from build123d import *

# Parameters (mm, degrees)
SKETCH_2_R      = 2.55
SKETCH_2_W      = 14
SKETCH_2_H      = 14
SKETCH_2_W_2    = 50
SKETCH_2_H_2    = 8
EXTRUDE_1_DEPTH = 5


with BuildPart() as part:
    # 草图2 → 凸台-拉伸1 (new body)
    with BuildSketch(Plane.XY):
        with BuildLine():
            Line((-130, 29.5), (130, 29.5))
            ThreePointArc((130, 29.5), (143.788582233, 23.788582233), (149.5, 10))
            Line((149.5, 10), (149.5, -110))
            ThreePointArc((149.5, -110), (143.788582233, -123.788582233), (130, -129.5))
            Line((130, -129.5), (-130, -129.5))
            ThreePointArc((-130, -129.5), (-143.788582233, -123.788582233), (-149.5, -110))
            Line((-149.5, -110), (-149.5, 10))
            ThreePointArc((-149.5, 10), (-143.788582233, 23.788582233), (-130, 29.5))
        make_face()
        with Locations((130, -110)):
            Circle(SKETCH_2_R, mode=Mode.SUBTRACT)
        with Locations((130, 10)):
            Circle(SKETCH_2_R, mode=Mode.SUBTRACT)
        with Locations((-130, -110)):
            Circle(SKETCH_2_R, mode=Mode.SUBTRACT)
        with Locations((-130, 10)):
            Circle(SKETCH_2_R, mode=Mode.SUBTRACT)
        with Locations((-61, -50)):
            Rectangle(SKETCH_2_W, SKETCH_2_H, mode=Mode.SUBTRACT)
        with Locations((-24, -50)):
            Rectangle(SKETCH_2_W, SKETCH_2_H, mode=Mode.SUBTRACT)
        with Locations((24, -50)):
            Rectangle(SKETCH_2_W, SKETCH_2_H, mode=Mode.SUBTRACT)
        with Locations((136, -87)):
            Rectangle(SKETCH_2_W, SKETCH_2_H, mode=Mode.SUBTRACT)
        with Locations((136, -13)):
            Rectangle(SKETCH_2_W, SKETCH_2_H, mode=Mode.SUBTRACT)
        with Locations((0, 6)):
            Rectangle(SKETCH_2_W_2, SKETCH_2_H_2, mode=Mode.SUBTRACT)
        with Locations((-136, -87)):
            Rectangle(SKETCH_2_W, SKETCH_2_H, mode=Mode.SUBTRACT)
        with Locations((-136, -13)):
            Rectangle(SKETCH_2_W, SKETCH_2_H, mode=Mode.SUBTRACT)
        with Locations((-98, -50)):
            Rectangle(SKETCH_2_W, SKETCH_2_H, mode=Mode.SUBTRACT)
        with Locations((61, -50)):
            Rectangle(SKETCH_2_W, SKETCH_2_H, mode=Mode.SUBTRACT)
        with Locations((98, -50)):
            Rectangle(SKETCH_2_W, SKETCH_2_H, mode=Mode.SUBTRACT)
        with BuildLine():
            Line((133.05, -25.838987573), (133.05, -30.161012427))
            ThreePointArc((133.05, -30.161012427), (132, -31.211012427), (130.95, -30.161012427))
            Line((130.95, -30.161012427), (130.95, -25.838987573))
            ThreePointArc((130.95, -25.838987573), (132, -24.788987573), (133.05, -25.838987573))
        make_face(mode=Mode.SUBTRACT)
        with BuildLine():
            Line((141.05, -26), (141.05, -30))
            ThreePointArc((141.05, -30), (140, -31.05), (138.95, -30))
            Line((138.95, -30), (138.95, -26))
            ThreePointArc((138.95, -26), (140, -24.95), (141.05, -26))
        make_face(mode=Mode.SUBTRACT)
        with BuildLine():
            Line((130.95, -74), (130.95, -70))
            ThreePointArc((130.95, -70), (132, -68.95), (133.05, -70))
            Line((133.05, -70), (133.05, -74))
            ThreePointArc((133.05, -74), (132, -75.05), (130.95, -74))
        make_face(mode=Mode.SUBTRACT)
        with BuildLine():
            Line((138.95, -74), (138.95, -70))
            ThreePointArc((138.95, -70), (140, -68.95), (141.05, -70))
            Line((141.05, -70), (141.05, -74))
            ThreePointArc((141.05, -74), (140, -75.05), (138.95, -74))
        make_face(mode=Mode.SUBTRACT)
        with BuildLine():
            Line((-141.05, -26), (-141.05, -30))
            ThreePointArc((-141.05, -30), (-140, -31.05), (-138.95, -30))
            Line((-138.95, -30), (-138.95, -26))
            ThreePointArc((-138.95, -26), (-140, -24.95), (-141.05, -26))
        make_face(mode=Mode.SUBTRACT)
        with BuildLine():
            Line((-133.05, -25.838987573), (-133.05, -30.161012427))
            ThreePointArc((-133.05, -30.161012427), (-132, -31.211012427), (-130.95, -30.161012427))
            Line((-130.95, -30.161012427), (-130.95, -25.838987573))
            ThreePointArc((-130.95, -25.838987573), (-132, -24.788987573), (-133.05, -25.838987573))
        make_face(mode=Mode.SUBTRACT)
        with BuildLine():
            Line((-130.95, -74), (-130.95, -70))
            ThreePointArc((-130.95, -70), (-132, -68.95), (-133.05, -70))
            Line((-133.05, -70), (-133.05, -74))
            ThreePointArc((-133.05, -74), (-132, -75.05), (-130.95, -74))
        make_face(mode=Mode.SUBTRACT)
        with BuildLine():
            Line((-138.95, -74), (-138.95, -70))
            ThreePointArc((-138.95, -70), (-140, -68.95), (-141.05, -70))
            Line((-141.05, -70), (-141.05, -74))
            ThreePointArc((-141.05, -74), (-140, -75.05), (-138.95, -74))
        make_face(mode=Mode.SUBTRACT)
        with BuildLine():
            Line((-62.5, -36.95), (-59.5, -36.95))
            ThreePointArc((-59.5, -36.95), (-58.45, -38), (-59.5, -39.05))
            Line((-59.5, -39.05), (-62.5, -39.05))
            ThreePointArc((-62.5, -39.05), (-63.55, -38), (-62.5, -36.95))
        make_face(mode=Mode.SUBTRACT)
        with BuildLine():
            Line((-62.5, -60.95), (-59.5, -60.95))
            ThreePointArc((-59.5, -60.95), (-58.45, -62), (-59.5, -63.05))
            Line((-59.5, -63.05), (-62.5, -63.05))
            ThreePointArc((-62.5, -63.05), (-63.55, -62), (-62.5, -60.95))
        make_face(mode=Mode.SUBTRACT)
        with BuildLine():
            Line((-15.5, -60.95), (-12.5, -60.95))
            ThreePointArc((-12.5, -60.95), (-11.45, -62), (-12.5, -63.05))
            Line((-12.5, -63.05), (-15.5, -63.05))
            ThreePointArc((-15.5, -63.05), (-16.55, -62), (-15.5, -60.95))
        make_face(mode=Mode.SUBTRACT)
        with BuildLine():
            Line((-12.5, -39.05), (-15.5, -39.05))
            ThreePointArc((-15.5, -39.05), (-16.55, -38), (-15.5, -36.95))
            Line((-15.5, -36.95), (-12.5, -36.95))
            ThreePointArc((-12.5, -36.95), (-11.45, -38), (-12.5, -39.05))
        make_face(mode=Mode.SUBTRACT)
        with BuildLine():
            Line((-109.5, -36.95), (-106.5, -36.95))
            ThreePointArc((-106.5, -36.95), (-105.45, -38), (-106.5, -39.05))
            Line((-106.5, -39.05), (-109.5, -39.05))
            ThreePointArc((-109.5, -39.05), (-110.55, -38), (-109.5, -36.95))
        make_face(mode=Mode.SUBTRACT)
        with BuildLine():
            Line((-109.5, -60.95), (-106.5, -60.95))
            ThreePointArc((-106.5, -60.95), (-105.45, -62), (-106.5, -63.05))
            Line((-106.5, -63.05), (-109.5, -63.05))
            ThreePointArc((-109.5, -63.05), (-110.55, -62), (-109.5, -60.95))
        make_face(mode=Mode.SUBTRACT)
        with BuildLine():
            Line((109.5, -36.95), (106.5, -36.95))
            ThreePointArc((106.5, -36.95), (105.45, -38), (106.5, -39.05))
            Line((106.5, -39.05), (109.5, -39.05))
            ThreePointArc((109.5, -39.05), (110.55, -38), (109.5, -36.95))
        make_face(mode=Mode.SUBTRACT)
        with BuildLine():
            Line((109.5, -60.95), (106.5, -60.95))
            ThreePointArc((106.5, -60.95), (105.45, -62), (106.5, -63.05))
            Line((106.5, -63.05), (109.5, -63.05))
            ThreePointArc((109.5, -63.05), (110.55, -62), (109.5, -60.95))
        make_face(mode=Mode.SUBTRACT)
        with BuildLine():
            Line((62.5, -60.95), (59.5, -60.95))
            ThreePointArc((59.5, -60.95), (58.45, -62), (59.5, -63.05))
            Line((59.5, -63.05), (62.5, -63.05))
            ThreePointArc((62.5, -63.05), (63.55, -62), (62.5, -60.95))
        make_face(mode=Mode.SUBTRACT)
        with BuildLine():
            Line((15.5, -60.95), (12.5, -60.95))
            ThreePointArc((12.5, -60.95), (11.45, -62), (12.5, -63.05))
            Line((12.5, -63.05), (15.5, -63.05))
            ThreePointArc((15.5, -63.05), (16.55, -62), (15.5, -60.95))
        make_face(mode=Mode.SUBTRACT)
        with BuildLine():
            Line((62.5, -36.95), (59.5, -36.95))
            ThreePointArc((59.5, -36.95), (58.45, -38), (59.5, -39.05))
            Line((59.5, -39.05), (62.5, -39.05))
            ThreePointArc((62.5, -39.05), (63.55, -38), (62.5, -36.95))
        make_face(mode=Mode.SUBTRACT)
        with BuildLine():
            Line((12.5, -39.05), (15.5, -39.05))
            ThreePointArc((15.5, -39.05), (16.55, -38), (15.5, -36.95))
            Line((15.5, -36.95), (12.5, -36.95))
            ThreePointArc((12.5, -36.95), (11.45, -38), (12.5, -39.05))
        make_face(mode=Mode.SUBTRACT)
    extrude(amount=EXTRUDE_1_DEPTH)


solid = part.part
Design review of the part built by this model. Coordinates are the model's own, in mm. Give positions to 0.01 mm unless a question says otherwise; leave off trailing zeros. Order: outer loops, then holes, each group sorted by start corner. A loop starts at its lowest first (then second) coordinate and runs counter-clockwise, first axis right, second up.
1. Add section C-C, the plane x = -3. State the section outline as (y, z) points, then the cut area to 3 significant figures.
Solution:
outline: (-129.5, 0) - (2, 0) - (2, 5) - (-129.5, 5) - close; (10, 0) - (29.5, 0) - (29.5, 5) - (10, 5) - close
area: 755 mm2
2. For pin 1 Ø1.5 at (x, z) = (134, 3) entering from -Y, flat-tipped, find the tip position at first contact; note if it passes through.
Solution:
pin 1: stops at y = -129.23
3. Add section A-A, the plane x = 102. State the section outline as (y, z) points, then the cut area to 3 significant figures.
Solution:
outline: (-129.5, 0) - (-57, 0) - (-57, 5) - (-129.5, 5) - close; (-43, 0) - (29.5, 0) - (29.5, 5) - (-43, 5) - close
area: 725 mm2
4. Mouldability with a two-part tool opening along X and no side actions: class faces 1 (the cylindrical face through (-127.57, -109.23, 2.46)), 2 (the flat face through (2, -49, 0)), 3 (the cylindrical face through (143.939, -123.636, 2.465)) as +X half, -X half, draft (parallel to the pull), parting line (faces both ways), or undercut.
Solution:
face 1: undercut
face 2: draft
face 3: +X half
5. Add section D-D, the plane z = 1.9. State how many separate pieces and enclosed holes the cut face has, then the cut area to 3 significant figures.
Solution:
separate pieces: 1
enclosed holes: 35
area: 44,600 mm2
6. Add section B-B, the plane y = -51. State the section outline as (x, z) points.
Solution:
outline: (-149.5, 0) - (-105, 0) - (-105, 5) - (-149.5, 5) - close; (-91, 0) - (-68, 0) - (-68, 5) - (-91, 5) - close; (-54, 0) - (-31, 0) - (-31, 5) - (-54, 5) - close; (-17, 0) - (17, 0) - (17, 5) - (-17, 5) - close; (31, 0) - (54, 0) - (54, 5) - (31, 5) - close; (68, 0) - (91, 0) - (91, 5) - (68, 5) - close; (105, 0) - (149.5, 0) - (149.5, 5) - (105, 5) - close
7. To check wall thickness, follow L1, parallel to Y at x = 130, z = 1.75; L2, parallel to X at y = -93.5, z = 1.55; L3, parallel to X at y = -71.5, z = 4.1. State the ranges of each line that lie inside material, in increasing order.
Solution:
L1: y = -129.5 to -112.55, -107.45 to -94, -80 to -20, -6 to 7.45, 12.55 to 29.5
L2: x = -149.5 to -143, -129 to 129, 143 to 149.5
L3: x = -149.5 to -141.05, -138.95 to -133.05, -130.95 to 130.95, 133.05 to 138.95, 141.05 to 149.5
